Autodesk Inventor part; units mm, degrees
ref_plane "YZ Plane" through (0, 0, 0) normal (1, 0, 0) x (0, 1, 0)
ref_plane "XZ Plane" through (0, 0, 0) normal (0, 1, 0) x (-1, 0, 0)
ref_plane "XY Plane" through (0, 0, 0) normal (0, 0, 1) x (1, 0, 0)
sketch "zaklad" plane through (0, 0, 0) normal (0, 0, 1) x (1, 0, 0)
  line L0 (0, 0) -> (109, 0)
  line L1 (109, 0) -> (109, -70)
  line L2 (109, -70) -> (0, -70)
  line L3 (0, -70) -> (0, 0)
  dimension "d0" = 109
  dimension "d1" = 70
extrude "Extrusion1" add sketch "zaklad" along normal blind 1.2 and the other way blind 0.4
sketch "uchyt_pro_desku" plane through (0, 0, 1.2) normal (0, 0, 1) x (1, 0, 0)
  line L0 (0, 0) -> (0, -70)
  line L1 (0, -35) -> (109, -35)
  line L2 (109, -70) -> (109, 0)
  circle A0 centre (17, -59) radius 4
  circle A1 centre (18, -11) radius 4
  circle A2 centre (92.9, -11) radius 4
  circle A3 centre (99, -59) radius 4
  dimension "d4" = 8
  dimension "d5" = 17
  dimension "d6" = 24
  dimension "d8" = 8
  dimension "d9" = 74.9
  dimension "d11" = 8
  dimension "d12" = 82
  dimension "d73" = 18
extrude "Extrusion2" add sketch "uchyt_pro_desku" along normal blind 7
sketch "stena_RJ45" plane through (0, 0, 1.2) normal (0, 0, 1) x (1, 0, 0)
  line L0 (-1.6, -15.7) -> (0, -15.7)
  line L1 (0, -15.7) -> (0, -32.5)
  line L2 (0, -32.5) -> (-1.6, -32.5)
  line L3 (-1.6, -32.5) -> (-1.6, -15.7)
  circle A0 centre (18, -11) radius 4
  line L4 (0, 0) -> (0, -70)
  dimension "d17" = 1.6
  dimension "d18" = 16.8
  dimension "d19" = 4.7
  dimension "d20" = 0
sketch "srouby_upevneni" plane through (0, 0, 1.2) normal (0, 0, 1) x (1, 0, 0)
  arc A0 (8, -66) -> (4, -62) centre (4, -66) ccw
  line L0 (0, -70) -> (109, -70)
  line L1 (0, 0) -> (0, -70)
  line L2 (8, -66) -> (8, -70)
  line L3 (4, -62) -> (0, -62)
  line L4 (0, -62) -> (0, -70)
  line L5 (8, -70) -> (0, -70)
  line L6 (109, -70) -> (109, 0)
  line L7 (109, -35) -> (0, -35)
  line L8 (54.5, -35) -> (54.5, -22.3833)
  arc A1 (4, -8) -> (8, -4) centre (4, -4) ccw
  line L9 (8, -4) -> (8, 0)
  line L10 (4, -8) -> (0, -8)
  line L11 (0, -8) -> (0, 0)
  line L12 (8, 0) -> (0, 0)
  arc A2 (105, -62) -> (101, -66) centre (105, -66) ccw
  line L13 (101, -66) -> (101, -70)
  line L14 (105, -62) -> (109, -62)
  line L15 (109, -62) -> (109, -70)
  line L16 (101, -70) -> (109, -70)
  line L17 (101, -4) -> (101, 0)
  arc A3 (101, -4) -> (105, -8) centre (105, -4) ccw
  line L18 (105, -8) -> (109, -8)
  line L19 (109, -8) -> (109, 0)
  line L20 (101, 0) -> (109, 0)
  dimension "d21" = 8
sketch "steny" plane through (0, 0, 1.2) normal (0, 0, 1) x (1, 0, 0)
  line L0 (0, -70) -> (109, -70)
  line L1 (109, -70) -> (109, 0)
  line L2 (109, 0) -> (0, 0)
  line L3 (0, 0) -> (0, -70)
  line L4 (0, -70) -> (0, -32.5)
  line L5 (0, -15.7) -> (0, 0)
  line L6 (0, -32.5) -> (-1.6, -32.5)
  line L7 (-1.6, -15.7) -> (0, -15.7)
  line L8 (-1.6, 1.6) -> (110.6, 1.6)
  line L9 (110.6, 1.6) -> (110.6, -71.6)
  line L10 (110.6, -71.6) -> (-1.6, -71.6)
  line L11 (-1.6, -71.6) -> (-1.6, -32.5)
  line L12 (-1.6, -15.7) -> (-1.6, 1.6)
  dimension "d74" = 1.6
extrude "Extrusion3" add sketch "steny" along normal blind 30.5 and the other way blind 1.6 contours L0 L1 L2 L3 L7 L12 L8 L9 L10 L11 L6
extrude "Extrusion4" add sketch "stena_RJ45" along normal blind 25.5 and the other way blind 1.6 contours L0 L1 L2 L3
extrude "Extrusion5" add sketch "srouby_upevneni" along normal blind 15 contours L2 L0 L1 L3 A0 | L1 L12 L9 A1 L10 | L18 A3 L17 L20 L6 | L13 A2 L14 L6 L0
sketch "diry" plane through (0, 0, 1.2) normal (0, 0, 1) x (1, 0, 0)
  arc A0 (8, -66) -> (4, -62) centre (4, -66) ccw
  arc A1 (4, -8) -> (8, -4) centre (4, -4) ccw
  arc A2 (101, -4) -> (105, -8) centre (105, -4) ccw
  arc A3 (105, -62) -> (101, -66) centre (105, -66) ccw
  point P0 (116, -66)
  point P1 (116, -66)
hole "Hole1" at (105, -66, 1.2) at (4, -4, 1.2) at (4, -66, 1.2) at (105, -4, 1.2) direction (0, 0, -1) diameter 2.55 end through all both
sketch "uchyt_pro_desku_diry" plane through (99, -59, 8.2) normal (0, 0, 1) x (1, 0, 0)
  circle A0 centre (0, 0) radius 4
  circle A1 centre (-82, 0) radius 4
  circle A2 centre (-81, 48) radius 4
  circle A3 centre (-6.1, 48) radius 4
  point P0 (-99, 59)
hole "Hole2" at (99, -59, 8.2) at (17, -59, 8.2) at (18, -11, 8.2) at (92.9, -11, 8.2) direction (0, 0, -1) diameter 3.3 depth 7 countersink diameter 3.75 countersink angle 10
sketch "dira_USB" plane through (-1.6, -71.9, -0.4) normal (-1, 0, 0) x (0, 0, 1)
  line L0 (16.6, 36.7) -> (10.6, 36.7)
  line L1 (10.6, 36.7) -> (10.6, 26.7)
  line L2 (10.6, 26.7) -> (16.6, 26.7)
  line L3 (16.6, 26.7) -> (16.6, 36.7)
  line L4 (27.1, 39.4) -> (32.1, 39.4)
  line L5 (0, 0.3) -> (0, 73.5)
  point P0 (0.4, 71.9)
  point P1 (0, 0)
  point P2 (0, 73.8)
  dimension "d60" = 6
  dimension "d61" = 10
  dimension "d62" = 2.7
  dimension "d63" = 10.6
extrude "Extrusion7" cut sketch "dira_USB" against normal blind 2
sketch "vyrez_napajeci_jack_nepouzivany" plane through (0, -70, 31.7) normal (1, 0, 0) x (0, 0, -1)
  line L0 (23.5, 21.8) -> (-6.5, 21.8)
  line L1 (-6.5, 21.8) -> (-6.5, 9.8)
  line L2 (-6.5, 9.8) -> (23.5, 9.8)
  line L3 (23.5, 9.8) -> (23.5, 21.8)
  line L4 (30.5, 62) -> (30.5, 8)
  line L5 (21.5, 24.8) -> (15.5, 24.8)
  point P0 (31.7, 70)
  dimension "d66" = 30
  dimension "d67" = 12
  dimension "d68" = 7
  dimension "d69" = 3
extrude "Extrusion8" cut sketch "vyrez_napajeci_jack_nepouzivany" against normal blind 0.5
fillet "Fillet1" radius 2 4 edges at (-1.6, -71.6, 15.65) (-1.6, 1.6, 15.65) (110.6, -71.6, 15.65) (110.6, 1.6, 15.65)
properties part number "case_bottom"
Source: CAD feature listing. Evaluate the final solid. Frame: model axes, mm. A direction names the side the tool comes from. Round coordinates to 2 decimals unless told otherwise and drop trailing zeros. Loops run counter-clockwise (first coordinate to the right, second up) from the corner with the lowest first, then second, coordinate; pieces in that order, holes last.
(1) Section query A-A (x = 92.9). Output: boundary loops of the cut face in (y, z) (3 decimals), and give its area (3 significant figures).
From the geometry:
outline: (-71.6, -0.4) - (1.6, -0.4) - (1.6, 31.7) - (0, 31.7) - (0, 1.2) - (-7, 1.2) - (-7, 8.2) - (-9.125, 8.2) - (-9.35, 5.628) - (-9.35, 1.2) - (-12.65, 1.2) - (-12.65, 5.628) - (-12.875, 8.2) - (-15, 8.2) - (-15, 1.2) - (-70, 1.2) - (-70, 31.7) - (-71.6, 31.7) - close
area: 247 mm2
(2) Access query for faces 5 (the flat face through (95, -12, 8.2)), 6 (the flat face through (54, 1.6, 15)). Directions: +Z, -Z, +X, -X, +Y, -Y. A direction counts if a zero-diameter tool reaches every point of the face in a straight line with its end or side. Return the directions, or none.
From the geometry:
face 5: +Z
face 6: +Z, -Z, +X, -X, +Y
(3) Pull-direction query (X, two-part tool) for faces 1 (the flat face through (105, -2, 16.2)), 2 (the flat face through (54, -34, -0.4)), 3 (the flat face through (101, -2, 9)), 4 (the flat face through (110.6, -35, 15)); classes: +X half, -X half, draft (parallel to the pull), parting line (faces both ways), or undercut.
From the geometry:
face 1: undercut
face 2: draft
face 3: undercut
face 4: +X half
(4) Section query C-C (z = 13.5). Give the number of separate pieces and of enclosed holes in the cut face, and give its area (3 significant figures).
From the geometry:
separate pieces: 1
enclosed holes: 4
area: 779 mm2
(5) Section query B-B (y = -11). Output: boundary loops of the cut face in (x, z) (3 decimals), and give its area (3 significant figures).
From the geometry:
outline: (-1.6, -0.4) - (110.6, -0.4) - (110.6, 31.7) - (109, 31.7) - (109, 1.2) - (96.9, 1.2) - (96.9, 8.2) - (94.775, 8.2) - (94.55, 5.628) - (94.55, 1.2) - (91.25, 1.2) - (91.25, 5.628) - (91.025, 8.2) - (88.9, 8.2) - (88.9, 1.2) - (22, 1.2) - (22, 8.2) - (19.875, 8.2) - (19.65, 5.628) - (19.65, 1.2) - (16.35, 1.2) - (16.35, 5.628) - (16.125, 8.2) - (14, 8.2) - (14, 1.2) - (0, 1.2) - (0, 31.7) - (-1.6, 31.7) - close
area: 342 mm2
(6) Material intervals for probe 1 along Y at (x, z) = (4, 5) (3 decimals); probe 2 along X at (y, z) = (-4, 7) (3 decimals); probe 3 along X at (y, z) = (-68, 3.5), sorted ascending.
From the geometry:
probe 1: y = -71.6 to -67.275, -64.725 to -62, -8 to -5.275, -2.725 to 1.6
probe 2: x = -1.6 to 2.725, 5.275 to 8, 101 to 103.725, 106.275 to 110.6
probe 3: x = -1.6 to 8, 101 to 110.6
(7) Contact query for flat-ended pins moving along their axis: pin 1 Ø2 at (x, y) = (92.9, -11) entering from +Z; pin 2 Ø1.3 at (x, z) = (-0.5, 30.5) entering from -Y; pin 3 Ø2.5 at (x, y) = (97, -60.5) entering from +Z; pin 4 Ø9 at (x, y) = (4.5, -2.5) entering from +Z. Output: stop coordinate, or through.
From the geometry:
pin 1: stops at z = 1.2
pin 2: stops at y = -71.58
pin 3: stops at z = 8.2
pin 4: stops at z = 31.7
(8) Section query D-D (x = 59). Output: boundary loops of the cut face in (y, z), and give its area (3 significant figures).
From the geometry:
outline: (-71.6, -0.4) - (1.6, -0.4) - (1.6, 31.7) - (0, 31.7) - (0, 1.2) - (-70, 1.2) - (-70, 31.7) - (-71.6, 31.7) - close
area: 215 mm2
